Can you work these out from the model? Positions are in its coordinate system, mm. Face numbers are marked on the shaded views. Coordinates: 2 decimals unless noted, no trailing zeros. Loops run counter-clockwise (first coordinate to the right, second up) from the corner with the lowest first, then second, coordinate; pieces in that order, holes last.
Autodesk Inventor part; units mm, degrees
ref_plane "YZ Plane" through (0, 0, 0) normal (1, 0, 0) x (0, 1, 0)
ref_plane "XZ Plane" through (0, 0, 0) normal (0, 1, 0) x (-1, 0, 0)
ref_plane "XY Plane" through (0, 0, 0) normal (0, 0, 1) x (1, 0, 0)
sketch "スケッチ1" plane through (0, 0, 0) normal (0, 0, 1) x (1, 0, 0)
  line L0 (0, 3.1754) -> (2.75, 1.5877)
  line L1 (2.75, 1.5877) -> (2.75, -1.5877)
  line L2 (2.75, -1.5877) -> (0, -3.1754)
  line L3 (0, -3.1754) -> (-2.75, -1.5877)
  line L4 (-2.75, -1.5877) -> (-2.75, 1.5877)
  line L5 (-2.75, 1.5877) -> (0, 3.1754)
  point P0 (0, 0)
  point P1 (0, 0)
  dimension "d0" = 5.5
extrude "押し出し1" add sketch "スケッチ1" along normal blind 3.5
sketch "スケッチ2" plane through (0, 0, 3.5) normal (0, 0, 1) x (1, 0, 0)
  circle A0 centre (0, 0) radius 2.75
extrude "押し出し2" add sketch "スケッチ2" along normal blind 0.8
sketch "スケッチ3" plane through (0, 0, 4.3) normal (0, 0, 1) x (1, 0, 0)
  circle A0 centre (0, 0) radius 1.5
  dimension "d5" = 3
extrude "押し出し3" cut sketch "スケッチ3" against normal through all
properties part number "ナイロンナットm3" material "鉄、可鍛鉄"
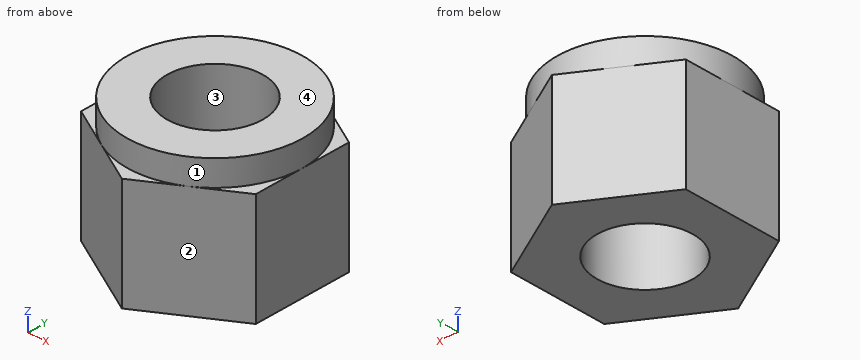
(1) If we mould it in two halves opening along X, with no side actions, what happens to the marked faces 1, 2, 3 and 4? For each: released by +X, released by -X, zero draft, split by the parting line, or undercut.
Check values:
face 1: split by the parting line
face 2: released by +X
face 3: undercut
face 4: zero draft
(2) I want a section at C-C on y = 1.75. Write out the boundary of the cut face in (x, z), then the cut area to 3 significant figures.
Check values:
outline: (-2.47, 0) - (2.47, 0) - (2.47, 3.5) - (2.12, 3.5) - (2.12, 4.3) - (-2.12, 4.3) - (-2.12, 3.5) - (-2.47, 3.5) - close
area: 20.7 mm2
(3) I'm going to push flat-ended pins straight in: pin 1 (1.5 mm diameter, centred on x = -2, z = 2.5, fed in from -Y); pin 2 (2.5 mm diameter, centred on x = 0, y = 0, fed in from -Z). Where does each tip first touch, or does it pass through?
Check values:
pin 1: stops at y = -2.45
pin 2: passes through
(4) If I drill on probe 1 along X at (y, z) = (0.25, 1.1); probe 2 along Y at (x, z) = (0.35, 3.8); probe 3 along Y at (x, z) = (-0.75, 4), over which ranges is the centre line in solid material (lowest first)?
Check values:
probe 1: x = -2.75 to -1.48, 1.48 to 2.75
probe 2: y = -2.73 to -1.46, 1.46 to 2.73
probe 3: y = -2.65 to -1.3, 1.3 to 2.65
(5) I want a section at D-D on x = 2.3. Write out the boundary of the cut face in (y, z).
Check values:
outline: (-1.85, 0) - (1.85, 0) - (1.85, 3.5) - (1.51, 3.5) - (1.51, 4.3) - (-1.51, 4.3) - (-1.51, 3.5) - (-1.85, 3.5) - close
(6) I want a section at A-A on z = 3.4. Write out the boundary of the cut face in (x, y), then the cut area to 3 significant figures.
Check values:
outline: (-2.75, -1.59) - (0, -3.18) - (2.75, -1.59) - (2.75, 1.59) - (0, 3.18) - (-2.75, 1.59) - close; hole circle Ø3 at (0, 0)
area: 19.1 mm2
